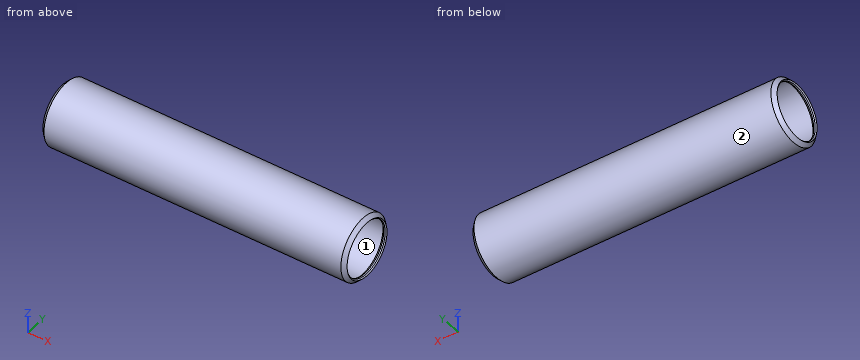
Autodesk Inventor part; units mm, degrees
ref_plane "o1_XY" through (0, -7.8105, 0) normal (1, 0, 0) x (0, 0, -1)
ref_plane "o1_YZ" through (0, -7.8105, 0) normal (0, 0, -1) x (0, 1, 0)
ref_plane "o1_ZX" through (0, -7.8105, 0) normal (0, 1, 0) x (1, 0, 0)
sketch "Sketch_5" plane through (0, 0, 0) normal (0, 0, 1) x (1, 0, 0)
  line L0 (76.2, 0) -> (-76.2, 0)
  line L1 (0, 6.9051) -> (0.263, 6.6421)
  line L2 (0.263, 6.6421) -> (0.635, 6.6421)
  line L3 (0.635, 6.6421) -> (1.27, 7.2771)
  line L4 (1.27, 7.2771) -> (74.93, 7.2771)
  line L5 (74.93, 7.2771) -> (75.565, 6.6421)
  line L6 (75.565, 6.6421) -> (75.937, 6.6421)
  line L7 (75.937, 6.6421) -> (76.2, 6.9051)
  line L8 (76.2, 6.9051) -> (75.2946, 7.8105)
  line L9 (75.2946, 7.8105) -> (0.9054, 7.8105)
  line L10 (0.9054, 7.8105) -> (0, 6.9051)
revolve "Revolution1" add sketch "Sketch_5" angle 360 about axis through (76.2, 0, 0) along (1, 0, 0)
ref_plane "o1_XY" through (0, -7.8105, 0) normal (1, 0, 0) x (0, 0, -1)
ref_plane "o1_YZ" through (0, -7.8105, 0) normal (0, 0, -1) x (0, 1, 0)
ref_plane "o1_ZX" through (0, -7.8105, 0) normal (0, 1, 0) x (1, 0, 0)
ref_plane "o2_XY" through (0, 7.8105, 0) normal (1, 0, 0) x (0, 0, -1)
ref_plane "o2_YZ" through (0, 7.8105, 0) normal (0, 0, -1) x (0, 1, 0)
ref_plane "o2_ZX" through (0, 7.8105, 0) normal (0, 1, 0) x (1, 0, 0)
ref_plane "t1_XY" through (38.1, 7.8105, 0) normal (1, 0, 0) x (0, 0, -1)
ref_plane "t1_YZ" through (38.1, 7.8105, 0) normal (0, 0, -1) x (0, 1, 0)
ref_plane "t1_ZX" through (38.1, 7.8105, 0) normal (0, 1, 0) x (1, 0, 0)
ref_plane "t2_XY" through (38.1, 0, -7.8105) normal (1, 0, 0) x (0, 0, -1)
ref_plane "t2_YZ" through (38.1, 0, -7.8105) normal (0, 0, -1) x (0, 1, 0)
ref_plane "t2_ZX" through (38.1, 0, -7.8105) normal (0, 1, 0) x (1, 0, 0)
ref_plane "t3_XY" through (38.1, -7.8105, 0) normal (1, 0, 0) x (0, 0, -1)
ref_plane "t3_YZ" through (38.1, -7.8105, 0) normal (0, 0, -1) x (0, 1, 0)
ref_plane "t3_ZX" through (38.1, -7.8105, 0) normal (0, 1, 0) x (1, 0, 0)
ref_plane "t4_XY" through (38.1, 0, 7.8105) normal (1, 0, 0) x (0, 0, -1)
ref_plane "t4_YZ" through (38.1, 0, 7.8105) normal (0, 0, -1) x (0, 1, 0)
ref_plane "t4_ZX" through (38.1, 0, 7.8105) normal (0, 1, 0) x (1, 0, 0)
ref_plane "tube1_XY" through (1.27, 0, 0) normal (1, 0, 0) x (0, 0, -1)
ref_plane "tube1_YZ" through (1.27, 0, 0) normal (0, 0, -1) x (0, 1, 0)
ref_plane "tube1_ZX" through (1.27, 0, 0) normal (0, 1, 0) x (1, 0, 0)
ref_plane "tube2_XY" through (74.93, 0, 0) normal (1, 0, 0) x (0, 0, -1)
ref_plane "tube2_YZ" through (74.93, 0, 0) normal (0, 0, -1) x (0, 1, 0)
ref_plane "tube2_ZX" through (74.93, 0, 0) normal (0, 1, 0) x (1, 0, 0)
properties part number "D-7516XP-3"
Verification items for the finished model (mm, model axes). Face numbers are marked on the shaded views. Give positions to 0.01 mm unless a question says otherwise; leave off trailing zeros. Order: outer loops, then holes, each group sorted by start corner. A loop starts at its lowest first (then second) coordinate and runs counter-clockwise, first axis right, second up. Notation, with made-up numbers: M 64.25,-12.5 L 85.25,-12.5 A20 ccw 85.25,-7.5 Z; hole C 11,2 d4. An arc over 180 degrees is marked long. Answer as a JSON object with one key per item and string values. Group by question number.
1) Cross-section at C-C (x = 51). Enter the section's corners in (y, z), then the cut area to 3 significant figures.
2) Depth check by flat-ended pin: pin 1 Ø2 at (x, y) = (68, -4.5) entering from +Z; pin 2 Ø6 at (x, y) = (65, 4) entering from +Z; pin 3 Ø1 at (x, z) = (11, 4) entering from +Y. Enter the tip coordinate at first touch or a pass-through.
3) Scan lines: line 1 along Y through (x, z) = (8.5, -0.25); line 2 along Z through (x, y) = (31, 0); line 3 along Y through (x, z) = (62.5, 4.75). Record each from-to range of solid material in increasing order. Write a range as [from, to].
4) Mould release check, pull along Y, two halves, no side actions. Record for the marked faces 1 and 2: released by +Y, released by -Y, zero draft, split by the parting line, or undercut.
Result sheet:
{
 "1": {"outline": "C 0,0 d15.62; hole C 0,0 d14.55", "area": "25.3 mm2"},
 "2": {"pin 1": "stops at z = 6.98", "pin 2": "stops at z = 7.75", "pin 3": "stops at y = 6.98"},
 "3": {"line 1": "y = [-7.81, -7.27], [7.27, 7.81]", "line 2": "z = [-7.81, -7.28], [7.28, 7.81]", "line 3": "y = [-6.2, -5.51], [5.51, 6.2]"},
 "4": {"face 1": "undercut", "face 2": "split by the parting line"}
}
